Autodesk Inventor part; units mm, degrees
ref_plane "YZ Plane" through (0, 0, 0) normal (1, 0, 0) x (0, 1, 0)
ref_plane "XZ Plane" through (0, 0, 0) normal (0, 1, 0) x (-1, 0, 0)
ref_plane "XY Plane" through (0, 0, 0) normal (0, 0, 1) x (1, 0, 0)
sketch "Sketch1" plane through (0, 0, 0) normal (1, 0, 0) x (0, 1, 0)
  circle A0 centre (0, 0) radius 22.5 construction
  circle A1 centre (0, 0) radius 16.25
  circle A2 centre (0, 0) radius 28.5
  circle A3 centre (15.9099, 15.9099) radius 2.65
  line L0 (15.9099, 15.9099) -> (0, 0) construction
  circle A4 centre (-15.9099, 15.9099) radius 2.65
  circle A5 centre (-15.9099, -15.9099) radius 2.65
  circle A6 centre (15.9099, -15.9099) radius 2.65
  line L1 (28.5, 0) -> (28.5, -38.5)
  line L2 (28.5, -38.5) -> (-28.5, -38.5)
  line L3 (-28.5, -38.5) -> (-28.5, 0)
  line L4 (28.5, -18.5) -> (-28.5, -18.5)
  line L5 (-28.5, -28.5) -> (-20.1554, -28.5) construction
  line L6 (-20.1554, -28.5) -> (-11.8108, -28.5) construction
  line L7 (20.1554, -28.5) -> (28.5, -28.5) construction
  circle A7 centre (20.1554, -28.5) radius 2.65
  circle A8 centre (-20.1554, -28.5) radius 2.65
  line L8 (0, 0) -> (0, 13.3225) construction
  line L9 (-28.5, -28.5) -> (-20.1554, -28.5) construction
  line L10 (20.1554, -28.5) -> (16.456, -23.2691) construction
  point P0 (-17.3108, 22.6404)
  point P1 (-26.3306, -10.9065)
  point P2 (28.5, 0)
  dimension "d0" = 45
  dimension "d1" = 32.5
  dimension "d2" = 57
  dimension "d3" = 5.3
  dimension "d6" = 360
  dimension "d12" = 20
  dimension "d22" = 5.3
  dimension "d23" = 10
  dimension "d24" = 45
  dimension "d27" = 10
  dimension "d28" = 8.3446
extrude "Extrusion1" add sketch "Sketch1" along normal blind 10 contours A2 L4 A6 A5 | L1 L4 A2 | A2 L4 L3 | L4 L1 L2 L3 A2 | A2 L4 A5 A6
fillet "Fillet1" radius 10 4 edges at (5, 28.5, -38.5) (5, -28.5, -38.5) (5, -28.5, 0) (5, 28.5, 0)
sketch "Sketch2" plane through (0, 0, 0) normal (-1, 0, 0) x (0, 0, 1)
  arc A0 (-38.5, -18.5) -> (-28.5, -28.5) centre (-28.5, -18.5) ccw
  line L0 (0, -28.5) -> (-28.5, -28.5)
  arc A1 (0, -28.5) -> (0, 28.5) centre (0, 0) ccw
  line L1 (-28.5, 28.5) -> (0, 28.5)
  arc A2 (-28.5, 28.5) -> (-38.5, 18.5) centre (-28.5, 18.5) ccw
  line L2 (-38.5, -18.5) -> (-38.5, 18.5)
  circle A3 centre (-28.5, 20.1554) radius 2.65
  circle A4 centre (-28.5, -20.1554) radius 2.65
  circle A5 centre (-15.9099, 15.9099) radius 2.65
  circle A6 centre (-15.9099, -15.9099) radius 2.65
  circle A7 centre (15.9099, -15.9099) radius 2.65
  circle A8 centre (15.9099, 15.9099) radius 2.65
  circle A9 centre (0, 0) radius 16.25
  circle A10 centre (-15.9099, 15.9099) radius 2.65
  circle A11 centre (-15.9099, 15.9099) radius 4.5
  circle A12 centre (-15.9099, -15.9099) radius 2.65
  circle A13 centre (-15.9099, -15.9099) radius 4.5
  circle A14 centre (15.9099, -15.9099) radius 2.65
  circle A15 centre (15.9099, -15.9099) radius 4.5
  circle A16 centre (15.9099, 15.9099) radius 2.65
  circle A17 centre (15.9099, 15.9099) radius 4.5
  dimension "d29" = 9
  dimension "d30" = 9
  dimension "d31" = 9
  dimension "d32" = 9
extrude "Extrusion2" cut sketch "Sketch2" against normal blind 5 contours A5 | A6 | A7 | A8 | A11 | A13 | A15 | A17
properties part number "Soporte motor"
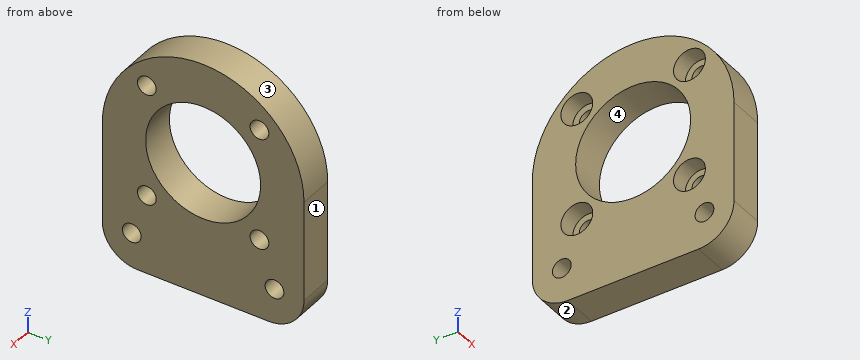
For this review, take the finished solid that the model builds, in its own axes (mm). Face numbers are marked on the shaded views. Round coordinates to 2 decimals unless told otherwise and drop trailing zeros. Order: outer loops, then holes, each group sorted by start corner. A loop starts at its lowest first (then second) coordinate and runs counter-clockwise, first axis right, second up.
Q1. Wall thickness on line 1 (Z direction, x = 4, y = -17); line 2 (Z direction, x = 4.25, y = 19); line 3 (Z direction, x = 1.25, y = -14): over which ranges is each line inside the solid? List them lowest first.
Findings below:
line 1: z = -38.5 to -20.28, -11.54 to 11.54, 20.28 to 22.87
line 2: z = -38.49 to -30.88, -26.12 to -19.18, -12.64 to 12.64, 19.18 to 21.24
line 3: z = -38.5 to -19.98, -11.84 to -8.25, 8.25 to 11.84, 19.98 to 24.82
Q2. We need section B-B, the plane z = 7. Give the boundary of the cut face in (x, y) (3 decimals), plus the area to 3 significant figures.
Findings below:
outline: (0, -27.627) - (10, -27.627) - (10, -14.665) - (0, -14.665) - close; (0, 14.665) - (10, 14.665) - (10, 27.627) - (0, 27.627) - close
area: 259 mm2
Q3. Insertion check: P1, Ø8, axis at y = -12, z = -1, coming from the -X side; P2, Ø7, axis at y = 15.91, z = -15.91, coming from the -X side; P3, Ø1.5, axis at x = 7.5, y = -3, coming from the +Z side. Each pin has a flat end and moves straight along its axis. Give the tip position at first contact, or say it passes through.
Findings below:
P1: passes through
P2: stops at x = 5
P3: stops at z = 28.41
Q4. We need section C-C, the plane x = 7. Give the boundary of the cut face in (y, z).
Findings below:
outline: (-28.5, -28.5) arc R10 ccw to (-18.5, -38.5) - (18.5, -38.5) arc R10 ccw to (28.5, -28.5) - (28.5, 0) arc R28.5 ccw to (-28.5, 0) - close; hole circle Ø5.3 at (-20.16, -28.5); hole circle Ø5.3 at (-15.91, -15.91); hole circle Ø5.3 at (-15.91, 15.91); hole circle Ø32.5 at (0, 0); hole circle Ø5.3 at (15.91, -15.91); hole circle Ø5.3 at (15.91, 15.91); hole circle Ø5.3 at (20.16, -28.5)
Q5. Mouldability with a two-part tool opening along Z and no side actions: class the marked faces 1, 2, 3 and 4 as pulls with the +Z half, pulls with the -Z half, needs draft (parallel to the pull), parting line crosses it, or undercut.
Findings below:
face 1: needs draft
face 2: pulls with the -Z half
face 3: pulls with the +Z half
face 4: undercut
Q6. We need section A-A, the plane y = 0. Give the boundary of the cut face in (x, z), plus the area to 3 significant figures.
Findings below:
outline: (0, -38.5) - (10, -38.5) - (10, -16.25) - (0, -16.25) - close; (0, 16.25) - (10, 16.25) - (10, 28.5) - (0, 28.5) - close
area: 345 mm2
